from build123d import *

# Parameters (mm, degrees)
ESBO_O1_R                = 2.5
RESSALTO_EXTRUS_O1_DEPTH = 3


with BuildPart() as part:
    # Esboço1 → Ressalto-extrusão1 (new body)
    with BuildSketch(Plane.XZ.offset(-10)):
        Polygon((-61.5, -9.199919627), (-61.5, -5), (-58.5, -5), (-58.5, 5), (-61.5, 5), (-61.5, 9.199919627), (-76.5, 9.199919627), (-76.5, 5), (-79.5, 5), (-79.5, -5), (-76.5, -5), (-76.5, -9.199919627), align=None)
        with Locations((-69, 0)):
            Circle(ESBO_O1_R, mode=Mode.SUBTRACT)
    extrude(amount=-RESSALTO_EXTRUS_O1_DEPTH)


solid = part.part
Read the model definition and answer for the solid it produces. Units are mm, in the model's axes. A direction names the side the tool comes from. Coordinates: 2 decimals unless noted, no trailing zeros. Order: outer loops, then holes, each group sorted by start corner. A loop starts at its lowest first (then second) coordinate and runs counter-clockwise, first axis right, second up. Notation, with made-up numbers: (19, 51.25) -> (26, 51.25) arc R13 ccw to (26, 72.25) -> close; hole circle Ø11 at (-30, -38). An arc over 180 degrees is marked (long way). Answer as a JSON object with one key per item and string values.
1) A cutting plane is placed at C-C, the plane z = 0. Determine the outline of the cut face in (x, y), plus the area to 3 significant figures.
Model answer:
{"outline": "(-79.5, 10) -> (-71.5, 10) -> (-71.5, 13) -> (-79.5, 13) -> close; (-66.5, 10) -> (-58.5, 10) -> (-58.5, 13) -> (-66.5, 13) -> close", "area": "48.0 mm²"}
2) A cutting plane is placed at A-A, the plane y = 11.4. Determine the outline of the cut face in (x, z).
Model answer:
{"outline": "(-79.5, -5) -> (-76.5, -5) -> (-76.5, -9.2) -> (-61.5, -9.2) -> (-61.5, -5) -> (-58.5, -5) -> (-58.5, 5) -> (-61.5, 5) -> (-61.5, 9.2) -> (-76.5, 9.2) -> (-76.5, 5) -> (-79.5, 5) -> close; hole circle Ø5 at (-69, 0)"}
3) A cutting plane is placed at B-B, the plane x = -69. Determine the outline of the cut face in (y, z), plus the area to 3 significant figures.
Model answer:
{"outline": "(10, -9.2) -> (13, -9.2) -> (13, -2.5) -> (10, -2.5) -> close; (10, 2.5) -> (13, 2.5) -> (13, 9.2) -> (10, 9.2) -> close", "area": "40.2 mm²"}
4) A tool of negligible diameter and unlimited length cuts with its end or side. For faces 5 (the face through (-78, 11, -5)), 6 (the face through (-60, 11, 5)), 7 (the face through (-78, 11, 5)), 8 (the face through (-60, 11, -5)), from which of +Z, -Z, +X, -X, +Y, -Y can it reach the whole face along a straight path? Write none if from no direction.
Model answer:
{"face 5": "-Z, -X, +Y, -Y", "face 6": "+Z, +X, +Y, -Y", "face 7": "+Z, -X, +Y, -Y", "face 8": "-Z, +X, +Y, -Y"}
5) Consider line 1 along Z through (x, y) = (-69, 12); line 2 along X through (y, z) = (11.95, 7.5); line 3 along Z through (x, y) = (-66.75, 12.65). Determine where each line is inside the solid, lowest interval first. Write a range as from..to.
Model answer:
{"line 1": "z = -9.2..-2.5, 2.5..9.2", "line 2": "x = -76.5..-61.5", "line 3": "z = -9.2..-1.09, 1.09..9.2"}
6) A cutting plane is placed at D-D, the plane z = -5.5. Determine the outline of the cut face in (x, y).
Model answer:
{"outline": "(-76.5, 10) -> (-61.5, 10) -> (-61.5, 13) -> (-76.5, 13) -> close"}
7) The mould has two halves that part along Z. Classify faces 1 (the face through (-69, 11, -9.2)), 2 (the face through (-71, 11.5, -1.5)), 3 (the face through (-69, 11, 9.2)), 4 (the face through (-61.5, 11, 7)): released by +Z, released by -Z, zero draft, split by the parting line, or undercut.
Model answer:
{"face 1": "released by -Z", "face 2": "undercut", "face 3": "released by +Z", "face 4": "zero draft"}
8) Each of these flat-tipped pins is pushed along its axis until it touches: pin 1 (1.5 mm diameter, centred on x = -78, y = 12, fed in from +Z); pin 2 (0.9 mm diameter, centred on y = 11.5, z = 6.5, fed in from -X); pin 3 (0.9 mm diameter, centred on x = -59.5, y = 12, fed in from -Z). Where does it stop, or does it pass through?
Model answer:
{"pin 1": "stops at z = 5", "pin 2": "stops at x = -76.5", "pin 3": "stops at z = -5"}
